Here's how the part is built. I have some questions about the finished solid (model axes, mm). A direction names the side the tool comes from. Coordinates: 2 decimals unless noted, no trailing zeros. Order: outer loops, then holes, each group sorted by start corner. A loop starts at its lowest first (then second) coordinate and runs counter-clockwise, first axis right, second up. Notation, with made-up numbers: (-17, -32.75) - (33, -32.75) arc R20 cw to (33, -0.75) - close; hole circle Ø9 at (-28.75, 36). An arc over 180 degrees is marked (long way). Answer in a Markdown table with one row per item. Add a question column.
Item 1: I want a section at C-C (x = -8). Please give me the cut outline in (y, z).
Item 2: I want a section at B-B (x = 50). Please give me the cut outline in (y, z).
Item 3: Thinking about a two-plate mould opening in X: for faces 4 (the flat face through (33, -11.782, 6)), 5 (the flat face through (7, -8, 9)), 6 (the cylindrical face through (-47.388, -7.684, 4.056)), 7 (the flat face through (61.757, -18, 4)), which applies, +X half, -X half, draft (parallel to the pull), parting line (faces both ways), or undercut?
Item 4: If I drill on line 1 along X through (y, z) = (-24, 5.5); line 2 along Z through (x, y) = (-34, -14.75); line 3 along Y through (x, z) = (20, 6.25), over which ranges is the centre line in solid material (lowest first)? Write a range as from..to.
Item 5: I want a section at D-D (x = -35.5). Please give me the cut outline in (y, z).
Item 6: Will these pins go through, and if not, where does the flat tip stop? pin 1 Ø1.5 at (x, z) = (21, 7.5) entering from -Y; pin 2 Ø5 at (x, y) = (-5, -22) entering from +Z.
Item 7: On a 3-axis mill with a long thin cutter (end or side, diameter ignored), from which of +Z, -Z, +X, -X, +Y, -Y can I reach the whole of each face in a straight line? I mean faces 1 (the flat face through (-33.633, -19.053, 1.26)), 2 (the flat face through (33, -19, 2)), 3 (the cylindrical face through (-36.677, -22.485, 0.254)). Say none if no direction works.
Item 8: I want a section at A-A (z = 4.75). Please give me the cut outline in (x, y), plus the area to 3 significant figures.
```python
from build123d import *

# Parameters (mm, degrees)
F0_W           = 110
F0_H           = 20
F1_DEPTH       = 9
F2_W           = 100
F2_H           = 15
F3_DEPTH       = 7
F4_R           = 3
F5_R           = 2
F6_DEPTH       = 20
F8_DEPTH       = 1.5
F9_R           = 9.25
F10_DEPTH      = 1.5
F10_DEPTH_BACK = 7
F11_R          = 1


with BuildPart() as f1:
    # F0 (on Top) → F1 (new body)
    with BuildSketch(Plane.XY):
        with Locations((6.7567551136, -16.7820947109)):
            Rectangle(F0_W, F0_H)
    extrude(amount=F1_DEPTH)

    # F2 (on face) → F3 (cut)
    with BuildSketch(Plane.XY.offset(9)):
        with Locations((6.7567551136, -19.2820947109)):
            Rectangle(F2_W, F2_H)
    extrude(amount=-F3_DEPTH, mode=Mode.SUBTRACT)

    # F4
    f4_edges = [f1.edges().sort_by_distance(p)[0] for p in [
        (-43.243245, -11.782095, 5.5),
        (56.756755, -11.782095, 5.5),
        (-48.243245, -6.782095, 4.5),
        (61.756755, -6.782095, 4.5),
    ]]
    fillet(f4_edges, radius=F4_R)

    # F5 (on face) → F6 (cut)
    with BuildSketch(Plane.XY.offset(2)):
        with Locations((49.7567551136, -20.5320947109)):
            Circle(F5_R)
        with Locations((-36.2432448864, -20.5320947109)):
            Circle(F5_R)
    extrude(amount=-F6_DEPTH, mode=Mode.SUBTRACT)

    # F7 (on face) → F8 (cut)
    with BuildSketch(Plane.XY.offset(2)):
        Polygon((-34.5111940788, -17.5320947109), (-37.975295694, -17.5320947109), (-39.7073465015, -20.5320947109), (-37.975295694, -23.5320947109), (-34.5111940788, -23.5320947109), (-32.7791432713, -20.5320947109), align=None)
        Polygon((53.2208567287, -20.5320947109), (51.4888059212, -17.5320947109), (48.024704306, -17.5320947109), (46.2926534985, -20.5320947109), (48.024704306, -23.5320947109), (51.4888059212, -23.5320947109), align=None)
    extrude(amount=-F8_DEPTH, mode=Mode.SUBTRACT)

    # F9 (on face) → F10 (cut, two sides)
    with BuildSketch(Plane.XY.offset(2)) as f10_sk:
        with Locations((6.7567551136, -18.2820947109)):
            Circle(F9_R)
    extrude(amount=-F10_DEPTH, mode=Mode.SUBTRACT)
    extrude(f10_sk.sketch, amount=F10_DEPTH_BACK, mode=Mode.SUBTRACT)

    # F11
    f11_edges = [f1.edges().sort_by_distance(p)[0] for p in [
        (6.756755, -6.782095, 9),
        (-48.243245, -26.782095, 4.5),
        (61.756755, -26.782095, 4.5),
        (59.256755, -26.782095, 9),
        (-45.743245, -26.782095, 9),
    ]]
    fillet(f11_edges, radius=F11_R)


solid = f1.part
```
Values follow:
| question | item | result |
|---|---|---|
| 1 | outline | (-26.78, 0) - (-6.78, 0) - (-6.78, 8) arc R1 ccw to (-7.78, 9) - (-11.78, 9) - (-11.78, 2) - (-26.78, 2) - close |
| 2 | outline | (-26.78, 0) - (-22.52, 0) - (-22.52, 0.5) - (-23.53, 0.5) - (-23.53, 2) - (-26.78, 2) - close; (-18.55, 0) - (-6.78, 0) - (-6.78, 8) arc R1 ccw to (-7.78, 9) - (-11.78, 9) - (-11.78, 2) - (-17.53, 2) - (-17.53, 0.5) - (-18.55, 0.5) - close |
| 3 | face 4 | undercut |
| 3 | face 5 | draft |
| 3 | face 6 | -X half |
| 3 | face 7 | +X half |
| 4 | line 1 | x = -48.24..-43.24, 56.76..61.76 |
| 4 | line 2 | z = 0..2 |
| 4 | line 3 | y = -11.78..-6.78 |
| 5 | outline | (-26.78, 0) - (-22.39, 0) - (-22.39, 0.5) - (-23.53, 0.5) - (-23.53, 2) - (-26.78, 2) - close; (-18.68, 0) - (-6.78, 0) - (-6.78, 8) arc R1 ccw to (-7.78, 9) - (-11.78, 9) - (-11.78, 2) - (-17.53, 2) - (-17.53, 0.5) - (-18.68, 0.5) - close |
| 6 | pin 1 | stops at y = -11.78 |
| 6 | pin 2 | stops at z = 2 |
| 7 | face 1 | +Z |
| 7 | face 2 | +Z, -Y |
| 7 | face 3 | +Z, -Z |
| 8 | outline | (-48.24, -25.78) arc R1 ccw to (-47.24, -26.78) - (-43.24, -26.78) - (-43.24, -14.78) arc R3 cw to (-40.24, -11.78) - (0.18, -11.78) arc R9.25 cw to (13.34, -11.78) - (53.76, -11.78) arc R3 cw to (56.76, -14.78) - (56.76, -26.78) - (60.76, -26.78) arc R1 ccw to (61.76, -25.78) - (61.76, -9.78) arc R3 ccw to (58.76, -6.78) - (-45.24, -6.78) arc R3 ccw to (-48.24, -9.78) - close |
| 8 | area | 675 mm^2 |
